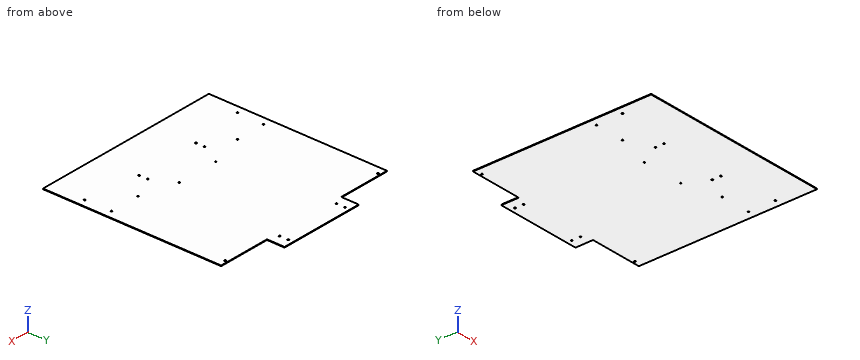
from build123d import *

# Parameters (mm, degrees)
BOSS_EXTRUDE1_DEPTH            = 3.175
F_1_4_CLEARANCE_HOLE1_D        = 6.7564
F_5_16_0_3125_DIAMETER_HOLE1_D = 7.9375


with BuildPart() as part:
    # Sketch2 → Boss-Extrude1 (new body)
    with BuildSketch(Plane.XY):
        Polygon((-482.6, 901.7), (-215.9, 901.7), (-215.9, 990.6), (215.9, 990.6), (215.9, 901.7), (482.6, 901.7), (482.6, 0), (-482.6, 0), align=None)
    extrude(amount=BOSS_EXTRUDE1_DEPTH)

    # 1/4 Clearance Hole1 (through all)
    with Locations(Plane.XY.offset(3.175)):
        with Locations((-441.96, 311.50918615), (105.907561142, 362.110143283), (289.91643105, 312.805115191), (-289.91643105, 312.805115191), (-105.907561142, 362.110143283), (441.96, 311.50918615)):
            Hole(F_1_4_CLEARANCE_HOLE1_D / 2)

    # 5/16 (0.3125) Diameter Hole1 (through all)
    with Locations(Plane.XY.offset(3.175)):
        with Locations((-165.1, 922.02), (-165.1, 965.2), (165.1, 965.2), (165.1, 922.02), (-165.1, 210.82), (-165.1, 254), (165.1, 254), (165.1, 210.82), (-444.5, 177.8), (444.5, 177.8), (-444.5, 889), (444.5, 889)):
            Hole(F_5_16_0_3125_DIAMETER_HOLE1_D / 2)


solid = part.part
The listing builds one solid part. Answer for the finished solid, in the listing's coordinates (mm). Give positions to 0.01 mm unless a question says otherwise; leave off trailing zeros. Write each loop counter-clockwise with the first axis right and the second up, starting at its lowest first coordinate (ties: lowest second). Pieces come first, ordered by that corner, then holes.
1) Section A-A (z = 1.4) is taken. Count the separate pieces of the cut face and the enclosed holes in it, and give its area (3 significant figures).
2) Given P1, Ø1, axis at x = 359, z = 2, coming from the +Y side; P2, Ø1, axis at y = 926.5, z = 1, coming from the +X side, each flat-ended and moving along its own axis, determine where each tip first touches the part or whether it passes through.
3) Section B-B (x = -308) is taken. Write down the section's boundary in (y, z) (3 decimals).
4) Find the intervals of material crossed by L1, parallel to Y at x = 165.1, z = 1.6; L2, parallel to X at y = 889, z = 1.3; L3, parallel to Y at x = 441.96, z = 2.1, in increasing order.
Response:
1. separate pieces: 1
1. enclosed holes: 18
1. area: 908,000 mm2
2. P1: stops at y = 901.7
2. P2: stops at x = 215.9
3. outline: (0, 0) - (901.7, 0) - (901.7, 3.175) - (0, 3.175) - close
4. L1: y = 0 to 206.85, 214.79 to 250.03, 257.97 to 918.05, 925.99 to 961.23, 969.17 to 990.6
4. L2: x = -482.6 to -448.47, -440.53 to 440.53, 448.47 to 482.6
4. L3: y = 0 to 174.75, 180.85 to 308.13, 314.89 to 885.95, 892.05 to 901.7
